from build123d import *
from build123d import SkipClean  # not in build123d's __all__

# Parameters (mm, degrees)
F0_R      = 6.35
F0_R_2    = 2.3876
F1_DEPTH  = 25.4
F2_W      = 25.4
F2_H      = 21.209
F3_DEPTH  = 2.3622
F4_R      = 7.874
F5_DEPTH  = 0.508
F6_R      = 2.3876
F7_DEPTH  = 28.2712
F8_R      = 3.937
F8_R_2    = 2.3876
F9_DEPTH  = 0.8636
F10_R     = 3.937
F11_DEPTH = 0.7874
F12_R     = 1.4732
F13_DEPTH = 3.7348


# Not quite as in the source:
# - after a boolean that leaves OpenCascade's solid faulty, fix() repairs it


with BuildPart() as f1:
    # F0 (on Front) → F1 (new body)
    with BuildSketch(Plane.XZ):
        Circle(F0_R)
        Circle(F0_R_2, mode=Mode.SUBTRACT)
    extrude(amount=F1_DEPTH)

    # F2 (on face) → F3 (join)
    with BuildSketch(Plane(origin=(0, 0, 0), x_dir=(-1, 0, 0), z_dir=(0, 1, 0))):
        Rectangle(F2_W, F2_H)
    extrude(amount=F3_DEPTH)

    # F4 (on face) → F5 (join)
    with BuildSketch(Plane(origin=(0, 2.3622, 0), x_dir=(-1, 0, 0), z_dir=(0, 1, 0))):
        Circle(F4_R)
    extrude(amount=F5_DEPTH)

    # F6 (on face) → F7 (cut, through all)
    with BuildSketch(Plane(origin=(0, 2.8702, 0), x_dir=(-1, 0, 0), z_dir=(0, 1, 0))):
        Circle(F6_R)
    with SkipClean():  # cleaning this boolean's faces spoils the solid; the shape is the same uncleaned
        extrude(amount=-F7_DEPTH, mode=Mode.SUBTRACT)

    # F8 (on face) → F9 (join)
    with BuildSketch(Plane(origin=(0, 2.8702, 0), x_dir=(-1, 0, 0), z_dir=(0, 1, 0))):
        Circle(F8_R)
        Circle(F8_R_2, mode=Mode.SUBTRACT)
    extrude(amount=F9_DEPTH)

    add(f1.part.fix(), mode=Mode.REPLACE)

    # F10 (on face) → F11 (join)
    with BuildSketch(Plane.XZ.offset(25.4)):
        Circle(F10_R)
        with BuildLine():
            ThreePointArc((2.3876, 0), (0, -2.3876), (-2.3876, 0))
            ThreePointArc((-2.3876, 0), (0, 2.3876), (2.3876, 0))
        make_face(mode=Mode.SUBTRACT)
    extrude(amount=F11_DEPTH)

    # F12 (on face) → F13 (cut, through all)
    with BuildSketch(Plane.XZ):
        with Locations((-10.414, 8.3185)):
            Circle(F12_R)
        with Locations((10.414, 8.3185)):
            Circle(F12_R)
        with Locations((-10.414, -8.3185)):
            Circle(F12_R)
        with Locations((10.414, -8.3185)):
            Circle(F12_R)
    extrude(amount=-F13_DEPTH, mode=Mode.SUBTRACT)


solid = f1.part
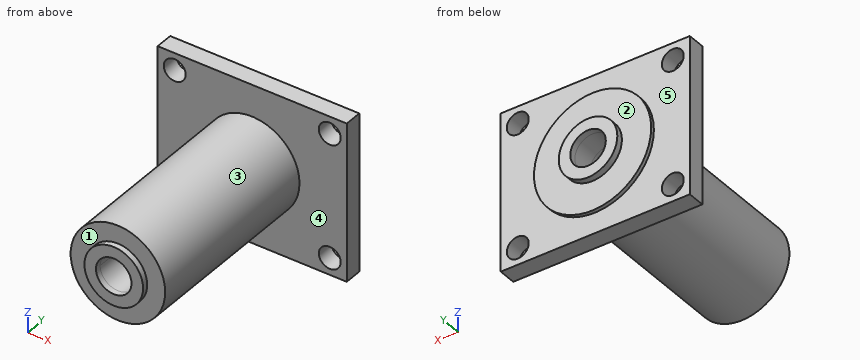
Source: CAD feature listing. Evaluate the final solid. Frame: model axes, mm. Face numbers are marked on the shaded views. A direction names the side the tool comes from. Coordinates: 2 decimals unless noted, no trailing zeros. Order: outer loops, then holes, each group sorted by start corner. A loop starts at its lowest first (then second) coordinate and runs counter-clockwise, first axis right, second up. Notation, with made-up numbers: M -1.75,39.5 L 27.25,39.5 A15 ccw 27.25,56.5 Z; hole C -20.75,69.5 d2. An arc over 180 degrees is marked long. Write each question's results on one line, items separated by ' | '. Start each with the question number.
1. Section A-A, the plane x = 0. Return the cut outline in (y, z).
2. Material intervals for L1, parallel to X at y = 0.25, z = -9; L2, parallel to Z at x = 0, y = 2.1; L3, parallel to Y at x = 5.25, z = -2.75, sorted ascending.
3. Reachability of the marked faces 4 and 5 from +Z, -Z, +X, -X, +Y, -Y: full face, straight path, thin tool, end or side. Return the list, or none.
4. Section D-D, the plane z = -5.75. Return the cut outline in (x, y).
5. Pin query (flat end, axial travel): pin 1 (6 mm diameter, centred on y = -19.5, z = -8.5, fed in from +X); pin 2 (2 mm diameter, centred on y = -8, z = -5, fed in from +X); pin 3 (5 mm diameter, centred on x = 8, z = 2.5, fed in from -Y); pin 4 (8 mm diameter, centred on x = -2, z = 0, fed in from +Y). Return the tip coordinate at first contact, or that it passes through.
6. Section C-C, the plane y = -14.75. Return the cut outline in (x, z), then the cut area to 3 significant figures.
7. Draft query along Y for the marked faces 1, 2 and 3. Return one class per face: +Y half, -Y half, draft (parallel to the pull), parting line (faces both ways), or undercut.
8. Section B-B, the plane x = -10.5. Return the cut outline in (y, z), then the cut area to 3 significant figures.
Solution:
1) outline: M -26.19,-3.94 L -25.4,-3.94 L -25.4,-6.35 L 0,-6.35 L 0,-10.6 L 2.36,-10.6 L 2.36,-7.87 L 2.87,-7.87 L 2.87,-3.94 L 3.73,-3.94 L 3.73,-2.39 L -26.19,-2.39 Z; M -26.19,2.39 L 3.73,2.39 L 3.73,3.94 L 2.87,3.94 L 2.87,7.87 L 2.36,7.87 L 2.36,10.6 L 0,10.6 L 0,6.35 L -25.4,6.35 L -25.4,3.94 L -26.19,3.94 Z
2) L1: -12.7 to -11.72, -9.11 to 9.11, 11.72 to 12.7 | L2: -10.6 to -2.39, 2.39 to 10.6 | L3: -25.4 to 2.87
3) face 4: -Y | face 5: +Y
4) outline: M -12.7,0 L -2.69,0 L -2.69,-25.4 L 2.69,-25.4 L 2.69,0 L 12.7,0 L 12.7,2.36 L 5.38,2.36 L 5.38,2.87 L -5.38,2.87 L -5.38,2.36 L -12.7,2.36 Z
5) pin 1: x = 3.17 | pin 2: x = 4.93 | pin 3: y = -25.4 | pin 4: y = 3.73
6) outline: C 0,0 d12.7; hole C 0,0 d4.78 | area: 109 mm²
7) face 1: -Y half | face 2: +Y half | face 3: draft
8) outline: M 0,-10.6 L 2.36,-10.6 L 2.36,-9.79 L 0,-9.79 Z; M 0,-6.85 L 2.36,-6.85 L 2.36,6.85 L 0,6.85 Z; M 0,9.79 L 2.36,9.79 L 2.36,10.6 L 0,10.6 Z | area: 36.2 mm²
